from build123d import *

# Parameters (mm, degrees)
BOX003_W          = 1.3
BOX003_H          = 3.3
BOX003_DEPTH      = 10
BOX002_W          = 1.3
BOX002_H          = 3.3
BOX002_DEPTH      = 10
CYLINDER004_R     = 1
CYLINDER004_DEPTH = 10
CYLINDER003_R     = 1
CYLINDER003_DEPTH = 10
CYLINDER001_R     = 5.5
CYLINDER001_DEPTH = 4
CYLINDER_R        = 5.9
CYLINDER_DEPTH    = 4
BOX001_W          = 20.5
BOX001_H          = 54.5
BOX001_DEPTH      = 2.5
BOX_W             = 20.5
BOX_H             = 40.7
BOX_DEPTH         = 38.5


with BuildPart() as cubo003:
    # Box003 → Box003 (new body)
    with BuildSketch(Plane(origin=(5.25, 46, 20), x_dir=(1, 0, 0), z_dir=(0, 0, 1))):
        with Locations((0.65, 1.65)):
            Rectangle(BOX003_W, BOX003_H)
    extrude(amount=BOX003_DEPTH)


with BuildPart() as obj1:
    # Box002 → Box002 (new body)
    with BuildSketch(Plane(origin=(5.25, -9, 20), x_dir=(1, 0, 0), z_dir=(0, 0, 1))):
        with Locations((0.65, 1.65)):
            Rectangle(BOX002_W, BOX002_H)
    extrude(amount=BOX002_DEPTH)

    # Fusion005: union Cubo003
    add(cubo003.part)


with BuildPart() as taladro2:
    # Cylinder004 → Cylinder004 (new body)
    with BuildSketch(Plane(origin=(5.9, 46.4, 21), x_dir=(1, 0, 0), z_dir=(0, 0, 1))):
        Circle(CYLINDER004_R)
    extrude(amount=CYLINDER004_DEPTH)


with BuildPart() as taladros001:
    # Cylinder003 → Cylinder003 (new body)
    with BuildSketch(Plane(origin=(5.9, -5.8, 21), x_dir=(1, 0, 0), z_dir=(0, 0, 1))):
        Circle(CYLINDER003_R)
    extrude(amount=CYLINDER003_DEPTH)

    # Fusion004: union Taladro2
    add(taladro2.part)

    # Fusion006: union obj1
    add(obj1.part)


with BuildPart() as cilindro001:
    # Cylinder001 → Cylinder001 (new body)
    with BuildSketch(Plane(origin=(9.9, 10.3, 37.7), x_dir=(1, 0, 0), z_dir=(0, 0, 1))):
        Circle(CYLINDER001_R)
    extrude(amount=CYLINDER001_DEPTH)


with BuildPart() as fusion001:
    # Cylinder → Cylinder (new body)
    with BuildSketch(Plane(origin=(9.9, 16.6, 37.7), x_dir=(1, 0, 0), z_dir=(0, 0, 1))):
        Circle(CYLINDER_R)
    extrude(amount=CYLINDER_DEPTH)

    # Fusion001: union Cilindro001
    add(cilindro001.part)


with BuildPart() as cubo001:
    # Box001 → Box001 (new body)
    with BuildSketch(Plane(origin=(0, -6.9, 26.6), x_dir=(1, 0, 0), z_dir=(0, 0, 1))):
        with Locations((10.25, 27.25)):
            Rectangle(BOX001_W, BOX001_H)
    extrude(amount=BOX001_DEPTH)


with BuildPart() as cuerpo_con_taladros:
    # Box → Box (new body)
    with BuildSketch(Plane.XY):
        with Locations((10.25, 20.35)):
            Rectangle(BOX_W, BOX_H)
    extrude(amount=BOX_DEPTH)

    # Fusion: union Cubo001
    add(cubo001.part)

    # Fusion003: union Fusion001
    add(fusion001.part)

    # Cut: cut Taladros001
    add(taladros001.part, mode=Mode.SUBTRACT)


with BuildPart() as cuerpo_con_taladros_1:
    # Cut placement: moved
    add(cuerpo_con_taladros.part.moved(Location((-5.9, 0, 0))))


solid = cuerpo_con_taladros_1.part
The listing builds one solid part. Answer for the finished solid, in the listing's coordinates (mm). A direction names the side the tool comes from. Give positions to 0.01 mm unless a question says otherwise; leave off trailing zeros. Write each loop counter-clockwise with the first axis right and the second up, starting at its lowest first coordinate (ties: lowest second). Pieces come first, ordered by that corner, then holes. Notation, with made-up numbers: (32, 52.5) -> (82, 52.5) arc R19 cw to (82, 83.5) -> close; hole circle Ø3 at (-4, 65). An arc over 180 degrees is marked (long way). Use a Markdown table: item, result.
(1) Section A-A, the plane y = 46.4 is taken. Determine the outline of the cut face in (x, z), then the cut area to 4 significant figures.
Return value:
| item | result |
|---|---|
| outline | (-5.9, 26.6) -> (-1, 26.6) -> (-1, 29.1) -> (-5.9, 29.1) -> close; (1, 26.6) -> (14.6, 26.6) -> (14.6, 29.1) -> (1, 29.1) -> close |
| area | 46.25 mm2 |
(2) Find the intervals of material crossed by probe 1 along X at (y, z) = (46.4, 27.8); probe 2 along Y at (x, z) = (8.75, 6); probe 3 along Z at (x, y) = (13.75, 6.5), in increasing order. Write a range as from..to.
Return value:
| item | result |
|---|---|
| probe 1 | -5.9..-1, 1..14.6 |
| probe 2 | 0..40.7 |
| probe 3 | 0..38.5 |
(3) Section B-B, the plane x = 4 is taken. Determine the outline of the cut face in (y, z), then the cut area to 3 significant figures.
Return value:
| item | result |
|---|---|
| outline | (-6.9, 26.6) -> (0, 26.6) -> (0, 0) -> (40.7, 0) -> (40.7, 26.6) -> (47.6, 26.6) -> (47.6, 29.1) -> (40.7, 29.1) -> (40.7, 38.5) -> (22.5, 38.5) -> (22.5, 41.7) -> (4.8, 41.7) -> (4.8, 38.5) -> (0, 38.5) -> (0, 29.1) -> (-6.9, 29.1) -> close |
| area | 1,660 mm2 |
(4) Flat-ended cylindrical pins translate along their axes: P1, Ø10, axis at x = -1.5, y = 24, coming from the +Z side; P2, Ø1, axis at x = -1, z = 12, coming from the +Y side; P3, Ø5, axis at x = 7.5, z = 35.5, coming from the -Y side; P4, Ø3.5, axis at x = 8.5, y = -3, coming from the +Z side. Find the tip coordinate at first contact, or state that the pin passes through.
Return value:
| item | result |
|---|---|
| P1 | z = 41.7 |
| P2 | y = 40.7 |
| P3 | y = 0 |
| P4 | z = 29.1 |
(5) Determine the mould class of faces 1 (the cylindrical face through (0, 45.4, 27.8)), 2 (the flat face through (4, -3, 29.1)), 3 (the flat face through (8, 47.6, 28)), 4 (the cylindrical face through (0, -4.8, 27.8)) for opening direction Y: released by +Y, released by -Y, zero draft, split by the parting line, or undercut.
Return value:
| item | result |
|---|---|
| face 1 | undercut |
| face 2 | zero draft |
| face 3 | released by +Y |
| face 4 | undercut |
(6) Section C-C, the plane y = 10.3 is taken. Determine the outline of the cut face in (x, z).
Return value:
| item | result |
|---|---|
| outline | (-5.9, 0) -> (14.6, 0) -> (14.6, 38.5) -> (9.5, 38.5) -> (9.5, 41.7) -> (-1.5, 41.7) -> (-1.5, 38.5) -> (-5.9, 38.5) -> close |
(7) Section D-D, the plane z = 16 is taken. Determine the outline of the cut face in (x, y).
Return value:
| item | result |
|---|---|
| outline | (-5.9, 0) -> (14.6, 0) -> (14.6, 40.7) -> (-5.9, 40.7) -> close |
(8) For faces 5 (the flat face through (4, -3, 26.6)), 6 (the flat face through (4, 44, 29.1)), 7 (the cylindrical face through (4.182, 22.497, 40.078)), determine the directions among +Z, -Z, +X, -X, +Y, -Y from which every point of the face is accessible in a straight line to the end or side of a thin tool.
Return value:
| item | result |
|---|---|
| face 5 | -Z, +X, -X, -Y |
| face 6 | +Z, +X, -X, +Y |
| face 7 | +Z |
